from build123d import *

# Parameters (mm, degrees)
F0_R     = 3.5
F0_R_2   = 4
F0_R_3   = 2.25
F1_DEPTH = 3
F2_DEPTH = 3.2


with BuildPart() as f1:
    # F0 (on Top) → F1 (new body)
    with BuildSketch(Plane.XY):
        Polygon((-1.795, -22.5), (-1.795, 9.1e-09), (-1.795, 22.5), (-71.98, 22.5), (-71.98, -22.5), align=None)
        with Locations((-67.98, -17.5)):
            Circle(F0_R, mode=Mode.SUBTRACT)
        with Locations((-31.99, 0)):
            Circle(F0_R_2, mode=Mode.SUBTRACT)
        with Locations((-67.98, 17.5)):
            Circle(F0_R, mode=Mode.SUBTRACT)
        Polygon((-1.795, 22.5), (-1.795, 9.1e-09), (-1.795, -22.5), (22.205, -22.5), (22.205, 22.5), align=None)
        with Locations((14.205, -17.5)):
            Circle(F0_R, mode=Mode.SUBTRACT)
        with BuildLine():
            ThreePointArc((-1.795, 9.1e-09), (6.2050000046, 8), (14.205, 0))
            ThreePointArc((14.205, 0), (6.2049999954, -8), (-1.795, 9.1e-09))
        make_face(mode=Mode.SUBTRACT)
        with Locations((14.205, 17.5)):
            Circle(F0_R, mode=Mode.SUBTRACT)
        with Locations((-67.98, 17.5)):
            Circle(F0_R)
        with Locations((-67.98, 17.5)):
            Circle(F0_R_3, mode=Mode.SUBTRACT)
        with Locations((-67.98, -17.5)):
            Circle(F0_R)
        with Locations((-67.98, -17.5)):
            Circle(F0_R_3, mode=Mode.SUBTRACT)
        with Locations((14.205, -17.5)):
            Circle(F0_R)
        with Locations((14.205, -17.5)):
            Circle(F0_R_3, mode=Mode.SUBTRACT)
        with Locations((14.205, 17.5)):
            Circle(F0_R)
        with Locations((14.205, 17.5)):
            Circle(F0_R_3, mode=Mode.SUBTRACT)
    extrude(amount=-F1_DEPTH)

    # F0 (on Top) → F2 (join)
    with BuildSketch(Plane.XY):
        with Locations((-67.98, 17.5)):
            Circle(F0_R)
        with Locations((-67.98, 17.5)):
            Circle(F0_R_3, mode=Mode.SUBTRACT)
        with Locations((-67.98, -17.5)):
            Circle(F0_R)
        with Locations((-67.98, -17.5)):
            Circle(F0_R_3, mode=Mode.SUBTRACT)
        with Locations((14.205, -17.5)):
            Circle(F0_R)
        with Locations((14.205, -17.5)):
            Circle(F0_R_3, mode=Mode.SUBTRACT)
        with Locations((14.205, 17.5)):
            Circle(F0_R)
        with Locations((14.205, 17.5)):
            Circle(F0_R_3, mode=Mode.SUBTRACT)
    extrude(amount=F2_DEPTH)


solid = f1.part
Geometry check sheet. Reference: the model listing, model coordinates, mm. A direction names the side the tool comes from. Give positions to 0.01 mm unless a question says otherwise; leave off trailing zeros. Order: outer loops, then holes, each group sorted by start corner. A loop starts at its lowest first (then second) coordinate and runs counter-clockwise, first axis right, second up.
1. Depth check by flat-ended pin: pin 1 (10.5 mm diameter, centred on x = -31.99, y = 0, fed in from +Z); pin 2 (3 mm diameter, centred on y = 14, z = 1, fed in from -X). Enter the tip coordinate at first touch or a pass-through.
Completed:
pin 1: stops at z = 0
pin 2: stops at x = -71.98
2. Sectioned sample at D-D (x = -67.98). Record the boundary of the cut face in (y, z), then the cut area to 3 significant figures.
Completed:
outline: (-22.5, -3) - (-19.75, -3) - (-19.75, 3.2) - (-21, 3.2) - (-21, 0) - (-22.5, 0) - close; (-15.25, -3) - (15.25, -3) - (15.25, 3.2) - (14, 3.2) - (14, 0) - (-14, 0) - (-14, 3.2) - (-15.25, 3.2) - close; (19.75, -3) - (22.5, -3) - (22.5, 0) - (21, 0) - (21, 3.2) - (19.75, 3.2) - close
area: 124 mm2
3. Sectioned sample at C-C (z = 2.25). Record the boundary of the cut face in (x, y) (3 decimals).
Completed:
outline: circle Ø7 at (-67.98, -17.5); circle Ø7 at (-67.98, 17.5); circle Ø7 at (14.205, -17.5); circle Ø7 at (14.205, 17.5); hole circle Ø4.5 at (-67.98, -17.5); hole circle Ø4.5 at (-67.98, 17.5); hole circle Ø4.5 at (14.205, -17.5); hole circle Ø4.5 at (14.205, 17.5)
4. Scan lines: line 1 (Y direction, x = -67.98, z = 1.8); line 2 (Y direction, x = 13, z = 2.5); line 3 (X direction, y = 16.5, z = -2) (3 decimals). Record each from-to range of solid material in increasing order.
Completed:
line 1: y = -21 to -19.75, -15.25 to -14, 14 to 15.25, 19.75 to 21
line 2: y = -20.79 to -19.4, -15.6 to -14.21, 14.21 to 15.6, 19.4 to 20.79
line 3: x = -71.98 to -69.996, -65.964 to 12.189, 16.221 to 22.205
5. Draft check along Y on faces 1 (the face through (-68.468, 15.304, 0.057)), 2 (the face through (14, 15, 3.2)), 3 (the face through (-26, -22.5, -1)). Enter one of: pulls with the +Y half, pulls with the -Y half, needs draft (parallel to the pull), parting line crosses it, or undercut.
Completed:
face 1: undercut
face 2: needs draft
face 3: pulls with the -Y half
6. Access from +Z, -Z, +X, -X, +Y, -Y to the whole of each face (thin tool, end or side, straight path). Record for faces 4 (the face through (13.75, -14.03, 1.58)), 5 (the face through (-68, 15, 3.2)).
Completed:
face 4: +Z
face 5: +Z, +X, -X, +Y, -Y
7. Sectioned sample at A-A (y = 17.5). Record the boundary of the cut face in (x, z) (3 decimals), then the cut area to 3 significant figures.
Completed:
outline: (-71.98, -3) - (-70.23, -3) - (-70.23, 3.2) - (-71.48, 3.2) - (-71.48, 0) - (-71.98, 0) - close; (-65.73, -3) - (11.955, -3) - (11.955, 3.2) - (10.705, 3.2) - (10.705, 0) - (-64.48, 0) - (-64.48, 3.2) - (-65.73, 3.2) - close; (16.455, -3) - (22.205, -3) - (22.205, 0) - (17.705, 0) - (17.705, 3.2) - (16.455, 3.2) - close
area: 272 mm2
8. Sectioned sample at B-B (x = -31.99). Record the boundary of the cut face in (y, z), then the cut area to 3 significant figures.
Completed:
outline: (-22.5, -3) - (-4, -3) - (-4, 0) - (-22.5, 0) - close; (4, -3) - (22.5, -3) - (22.5, 0) - (4, 0) - close
area: 111 mm2
